```python
from build123d import *

# Parameters (mm, degrees)
SKETCH20_W                           = 44.45
SKETCH20_H                           = 21.59
BOSS_EXTRUDE3_DEPTH                  = 25.4
SKETCH22_W                           = 44.45
SKETCH22_H                           = 2.413
CUT_EXTRUDE2_DEPTH                   = 25.4
SKETCH23_W                           = 44.45
SKETCH23_H                           = 2.54
CUT_EXTRUDE3_DEPTH                   = 25.4
F_4_0_209_DIAMETER_HOLE6_D           = 5.3086
F_4_0_209_DIAMETER_HOLE6_CSINK_D     = 6.5786
F_4_0_209_DIAMETER_HOLE6_CSINK_ANGLE = 90
F_4_0_209_DIAMETER_HOLE7_D           = 5.3086
F_4_0_209_DIAMETER_HOLE7_CSINK_D     = 6.5786
F_4_0_209_DIAMETER_HOLE7_CSINK_ANGLE = 90


with BuildPart() as part:
    # Loft1: read off the stored shape, not the designer's step
    # Loft1: loft between two sections, ruled curve by curve
    loft1_from = [
        Edge.make_bspline([(-73.025, 50.8, -73.025), (-48.683333333, 50.8, -73.025), (-24.341666667, 50.8, -73.025), (24.341666667, 50.8, -73.025), (48.683333333, 50.8, -73.025), (73.025, 50.8, -73.025)], [0, 0, 0, 0, 0.5, 0.5, 1, 1, 1, 1], 3),
        Edge.make_bspline([(73.025, 50.8, -73.025), (73.025, 50.8, -48.683333333), (73.025, 50.8, -24.341666667), (73.025, 50.8, 24.341666667), (73.025, 50.8, 48.683333333), (73.025, 50.8, 73.025)], [0, 0, 0, 0, 0.5, 0.5, 1, 1, 1, 1], 3),
        Edge.make_bspline([(-73.025, 50.8, 73.025), (-73.025, 50.8, 48.683333333), (-73.025, 50.8, 24.341666667), (-73.025, 50.8, -24.341666667), (-73.025, 50.8, -48.683333333), (-73.025, 50.8, -73.025)], [0, 0, 0, 0, 0.5, 0.5, 1, 1, 1, 1], 3),
        Edge.make_bspline([(73.025, 50.8, 73.025), (48.683333333, 50.8, 73.025), (24.341666667, 50.8, 73.025), (-24.341666667, 50.8, 73.025), (-48.683333333, 50.8, 73.025), (-73.025, 50.8, 73.025)], [0, 0, 0, 0, 0.5, 0.5, 1, 1, 1, 1], 3),
    ]
    loft1_to = [
        Edge.make_bspline([(-76.2, 0, 76.2), (-76.2, 0, 50.8), (-76.2, 0, 25.4), (-76.2, 0, -25.4), (-76.2, 0, -50.8), (-76.2, 0, -76.2)], [0, 0, 0, 0, 0.5, 0.5, 1, 1, 1, 1], 3),
        Edge.make_bspline([(-76.2, 0, -76.2), (-50.8, 0, -76.2), (-25.4, 0, -76.2), (25.4, 0, -76.2), (50.8, 0, -76.2), (76.2, 0, -76.2)], [0, 0, 0, 0, 0.5, 0.5, 1, 1, 1, 1], 3),
        Edge.make_bspline([(76.2, 0, 76.2), (50.8, 0, 76.2), (25.4, 0, 76.2), (-25.4, 0, 76.2), (-50.8, 0, 76.2), (-76.2, 0, 76.2)], [0, 0, 0, 0, 0.5, 0.5, 1, 1, 1, 1], 3),
        Edge.make_bspline([(76.2, 0, -76.2), (76.2, 0, -50.8), (76.2, 0, -25.4), (76.2, 0, 25.4), (76.2, 0, 50.8), (76.2, 0, 76.2)], [0, 0, 0, 0, 0.5, 0.5, 1, 1, 1, 1], 3),
    ]
    loft1 = Solid(Shell([*[Face.make_surface_from_curves(loft1_from[k], loft1_to[k]) for k in range(4)], Face(Wire(loft1_from)), Face(Wire(loft1_to))]))
    add(loft1)

    # Sketch20 → Boss-Extrude3 (add)
    with BuildSketch(Plane(origin=(0, 50.8, 0), x_dir=(1, 0, 0), z_dir=(0, 1, 0))):
        with Locations((-50.8, -62.23)):
            Rectangle(SKETCH20_W, SKETCH20_H)
        with Locations((50.8, 62.23)):
            Rectangle(SKETCH20_W, SKETCH20_H)
    extrude(amount=BOSS_EXTRUDE3_DEPTH)

    # Sketch22 → Cut-Extrude2 (cut)
    with BuildSketch(Plane(origin=(0, 76.2, 0), x_dir=(1, 0, 0), z_dir=(0, 1, 0))):
        with Locations((-50.8, -62.1665)):
            Rectangle(SKETCH22_W, SKETCH22_H)
    extrude(amount=-CUT_EXTRUDE2_DEPTH, mode=Mode.SUBTRACT)

    # Sketch23 → Cut-Extrude3 (cut)
    with BuildSketch(Plane(origin=(0, 76.2, 0), x_dir=(1, 0, 0), z_dir=(0, 1, 0))):
        with Locations((50.8, 64.77)):
            Rectangle(SKETCH23_W, SKETCH23_H)
    extrude(amount=-CUT_EXTRUDE3_DEPTH, mode=Mode.SUBTRACT)

    # #4 (0.209) Diameter Hole6 (through all)
    with Locations(Plane.XY.offset(73.025)):
        with Locations((-51.435, 63.246)):
            CounterSinkHole(F_4_0_209_DIAMETER_HOLE6_D / 2, F_4_0_209_DIAMETER_HOLE6_CSINK_D / 2, counter_sink_angle=F_4_0_209_DIAMETER_HOLE6_CSINK_ANGLE)

    # #4 (0.209) Diameter Hole7 (through all)
    with Locations(Plane.XY.offset(-51.435)):
        with Locations((50.165, 63.246)):
            CounterSinkHole(F_4_0_209_DIAMETER_HOLE7_D / 2, F_4_0_209_DIAMETER_HOLE7_CSINK_D / 2, counter_sink_angle=F_4_0_209_DIAMETER_HOLE7_CSINK_ANGLE)


solid = part.part
```
The model under review builds one solid part; all positions refer to its coordinate system, in mm. A direction names the side the tool comes from. Coordinates: 2 decimals unless noted, no trailing zeros. Write each loop counter-clockwise with the first axis right and the second up, starting at its lowest first coordinate (ties: lowest second). Pieces come first, ordered by that corner, then holes. Notation, with made-up numbers: (-26.75, -25) - (6.25, -25) arc R6 cw to (6.25, -15) - close; hole circle Ø8 at (-18.75, 55). An arc over 180 degrees is marked (long way). Write item = value, one per line.
(1) Mouldability with a two-part tool opening along Y and no side actions: class faces 1 (the face through (-51, 76.2, 68)), 2 (the face through (-56, 63, 73.025)), 3 (the face through (48.738, 65.484, -57.865)) as pulls with the +Y half, pulls with the -Y half, needs draft (parallel to the pull), parting line crosses it, or undercut.
Result sheet:
face_1 = pulls with the +Y half
face_2 = needs draft
face_3 = undercut
(2) For P1, Ø8.5, axis at x = -51.435, y = 63.246, coming from the +Z side (3 decimals); P2, Ø10.5, axis at y = 57.5, z = 68.5, coming from the +X side (3 decimals); P3, Ø1, axis at x = -21.5, z = -16.5, coming from the +Y side; P4, Ø5, axis at x = 50.165, y = 63.246, coming from the -Z side, all flat-tipped, find the tip position at first contact; note any pin that passes through.
Result sheet:
P1 = 73.025
P2 = -28.575
P3 = 50.8
P4 = through
(3) For line 1 (Z direction, x = 29, y = 53) (3 decimals); line 2 (Y direction, x = -66.5, z = 2); line 3 (Y direction, x = 3.5, z = 34.5), list the stretches that pass through material, from the lowest coordinate up. Write a range as [from, to].
Result sheet:
line_1 = [-73.025, -66.04], [-63.5, -51.435]
line_2 = [0, 8.13], [21.05, 28.58], [45.83, 50.8]
line_3 = [0, 50.8]
(4) Machinability: for faces 4 (the face through (-51, 67, 60.96)), 5 (the face through (-51.1, 66.1, 51.435)), 6 (the face through (55, 63, -51.435)), 7 (the face through (-73.025, 63, 56)), 8 (the face through (-28.575, 63, 68)), which of the approach directions +Z, -Z, +X, -X, +Y, -Y give a long, thin tool a straight path to every point of the face, cutting with its end or side? Answer none if there is none.
Result sheet:
face_4 = +X, -X, +Y
face_5 = -Z, +X, -X, +Y
face_6 = +Z, +X, -X, +Y
face_7 = +Z, -Z, -X, +Y
face_8 = +Z, -Z, +X, +Y
(5) Consider section A-A, the plane y = 70. Give the boundary of the cut face in (x, z) (3 decimals), then the cut area to 3 significant figures.
Result sheet:
outline = (-73.025, 51.435) - (-28.575, 51.435) - (-28.575, 60.96) - (-73.025, 60.96) - close; (-73.025, 63.373) - (-28.575, 63.373) - (-28.575, 73.025) - (-73.025, 73.025) - close; (28.575, -73.025) - (73.025, -73.025) - (73.025, -66.04) - (28.575, -66.04) - close; (28.575, -63.5) - (73.025, -63.5) - (73.025, -51.435) - (28.575, -51.435) - close
area = 1,700 mm^2
